Input: part model. Units: mm. Frame: model coordinates. Face numbers are marked on the shaded views. A direction names the side the tool comes from. Round coordinates to 2 decimals unless told otherwise and drop trailing zeros. Loops run counter-clockwise (first coordinate to the right, second up) from the corner with the lowest first, then second, coordinate; pieces in that order, holes last. Notation, with made-up numbers: (88.25, -4) - (119.25, -4) arc R16 ccw to (119.25, 17) - close; hole circle Ø1 at (29, 45). An arc over 180 degrees is marked (long way). Write each question's results on one line, items separated by ' | '.
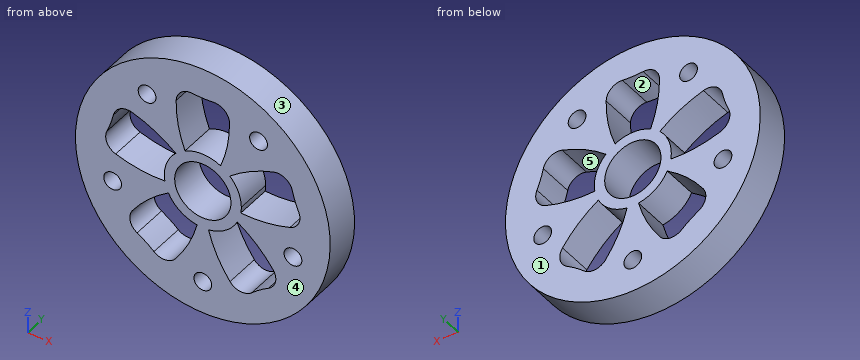
from build123d import *

# Parameters (mm, degrees)
SKETCH_1_R               = 43
SKETCH_1_R_2             = 9.5
SKETCH_1_R_3             = 3
EXTRUDE_1_DEPTH          = 12
CUT_EXTRUDE_1_DEPTH      = 62.983868869
CUT_EXTRUDE_1_DEPTH_BACK = 62.983868869


with BuildPart() as part:
    # 草图1 → 凸台-拉伸1 (new body)
    with BuildSketch(Plane(origin=(0, 0, 0), x_dir=(1, 0, 0), z_dir=(0, 1, 0))):
        with Locations(Location((0, 0, 0), (0, 0, 270))):
            Circle(SKETCH_1_R)
        with Locations(Location((0, 0, 0), (0, 0, 270))):
            Circle(SKETCH_1_R_2, mode=Mode.SUBTRACT)
        with Locations(Location((0, 32, 0), (0, 0, 270))):
            Circle(SKETCH_1_R_3, mode=Mode.SUBTRACT)
        with Locations(Location((30.433808521, 9.88854382, 0), (0, 0, 270))):
            Circle(SKETCH_1_R_3, mode=Mode.SUBTRACT)
        with Locations(Location((18.809128073, -25.88854382, 0), (0, 0, 270))):
            Circle(SKETCH_1_R_3, mode=Mode.SUBTRACT)
        with Locations(Location((-18.809128073, -25.88854382, 0), (0, 0, 270))):
            Circle(SKETCH_1_R_3, mode=Mode.SUBTRACT)
        with Locations(Location((-30.433808521, 9.88854382, 0), (0, 0, 270))):
            Circle(SKETCH_1_R_3, mode=Mode.SUBTRACT)
    extrude(amount=EXTRUDE_1_DEPTH)

    # 草图2 → 切除-拉伸1 (cut, two sides: drawn at the far end of the back side and taken through both)
    with BuildSketch(Plane(origin=(0, 0, 0), x_dir=(1, 0, 0), z_dir=(0, 1, 0)).offset(-CUT_EXTRUDE_1_DEPTH_BACK)):
        with BuildLine():
            ThreePointArc((-23.848620344, -17.211397152), (-16.091180112, -13.964625454), (-9.114016839, -9.270096928))
            ThreePointArc((-9.114016839, -9.270096928), (-12.363734712, -4.017220927), (-12.822220771, 2.142581267))
            ThreePointArc((-12.822220771, 2.142581267), (-21.226239066, 1.839460951), (-29.410544568, -0.093554533))
            ThreePointArc((-29.410544568, -0.093554533), (-32.369922784, -2.815813731), (-32.36785177, -6.83683478))
            ThreePointArc((-32.36785177, -6.83683478), (-31.119439219, -10.111318738), (-30.204732809, -13.494230394))
            ThreePointArc((-30.204732809, -13.494230394), (-27.842911423, -16.748522069), (-23.848620344, -17.211397152))
        make_face()
        with BuildLine():
            ThreePointArc((8.999382438, -28), (8.308699922, -19.618928286), (6, -11.532562595))
            ThreePointArc((6, -11.532562595), (0, -13), (-6, -11.532562595))
            ThreePointArc((-6, -11.532562595), (-8.308699922, -19.618928286), (-8.999382438, -28))
            ThreePointArc((-8.999382438, -28), (-7.324858249, -31.655760291), (-3.5, -32.896354479))
            ThreePointArc((-3.5, -32.896354479), (0, -32.720914778), (3.5, -32.896354479))
            ThreePointArc((3.5, -32.896354479), (7.324858249, -31.655760291), (8.999382438, -28))
        make_face()
        with BuildLine():
            ThreePointArc((12.822220771, 2.142581267), (12.955478957, 1.074972086), (13, 0))
            ThreePointArc((13, 0), (11.989208041, -5.025822375), (9.114016839, -9.270096928))
            ThreePointArc((9.114016839, -9.270096928), (16.091180112, -13.964625454), (23.848620344, -17.211397152))
            ThreePointArc((23.848620344, -17.211397152), (27.842911423, -16.748522069), (30.204732809, -13.494230394))
            ThreePointArc((30.204732809, -13.494230394), (31.119439219, -10.111318738), (32.36785177, -6.83683478))
            ThreePointArc((32.36785177, -6.83683478), (32.369922784, -2.815813731), (29.410544568, -0.093554533))
            ThreePointArc((29.410544568, -0.093554533), (21.226239066, 1.839460951), (12.822220771, 2.142581267))
        make_face()
        with BuildLine():
            ThreePointArc((1.924568248, 12.856750642), (7.64120828, 10.517220927), (11.632772181, 5.803327614))
            ThreePointArc((11.632772181, 5.803327614), (18.25359615, 10.988315115), (23.738640395, 17.362771566))
            ThreePointArc((23.738640395, 17.362771566), (24.532723854, 21.304604391), (22.167551497, 24.556461444))
            ThreePointArc((22.167551497, 24.556461444), (19.232871148, 26.471776127), (16.504432537, 28.67095821))
            ThreePointArc((16.504432537, 28.67095821), (12.680854244, 29.915491699), (9.177333733, 27.942180119))
            ThreePointArc((9.177333733, 27.942180119), (4.809837274, 20.755777674), (1.924568248, 12.856750642))
        make_face()
        with BuildLine():
            ThreePointArc((-11.632772181, 5.803327614), (-7.64120828, 10.517220927), (-1.924568248, 12.856750642))
            ThreePointArc((-1.924568248, 12.856750642), (-4.809837274, 20.755777674), (-9.177333733, 27.942180119))
            ThreePointArc((-9.177333733, 27.942180119), (-12.680854244, 29.915491699), (-16.504432537, 28.67095821))
            ThreePointArc((-16.504432537, 28.67095821), (-19.232871148, 26.471776127), (-22.167551497, 24.556461444))
            ThreePointArc((-22.167551497, 24.556461444), (-24.532723854, 21.304604391), (-23.738640395, 17.362771566))
            ThreePointArc((-23.738640395, 17.362771566), (-18.25359615, 10.988315115), (-11.632772181, 5.803327614))
        make_face()
    extrude(amount=CUT_EXTRUDE_1_DEPTH + CUT_EXTRUDE_1_DEPTH_BACK, mode=Mode.SUBTRACT)


solid = part.part
1. Section query C-C, the plane z = 16. Output: boundary loops of the cut face in (x, y).
Answer:
outline: (-39.91, 0) - (-28.82, 0) - (-28.82, 12) - (-39.91, 12) - close; (-20.43, 0) - (-7.49, 0) - (-7.49, 12) - (-20.43, 12) - close; (7.49, 0) - (20.43, 0) - (20.43, 12) - (7.49, 12) - close; (28.82, 0) - (39.91, 0) - (39.91, 12) - (28.82, 12) - close
2. Section query A-A, the plane x = 0. Output: boundary loops of the cut face in (y, z).
Answer:
outline: (0, -43) - (12, -43) - (12, -35) - (0, -35) - close; (0, -29) - (12, -29) - (12, -9.5) - (0, -9.5) - close; (0, 9.5) - (12, 9.5) - (12, 13) - (0, 13) - close; (0, 32.72) - (12, 32.72) - (12, 43) - (0, 43) - close
3. Set-up query: the marked faces 1 and 2. Return all of +Z, -Z, +X, -X, +Y, -Y with unobstructed straight access to the full face (end or side cutting, diameter ignored); none if empty.
Answer:
face 1: +Z, -Z, +X, -X, +Y | face 2: +Y, -Y
4. Mould query, pull axis X, two halves, no side actions, for the marked faces 3, 4 and 5. Classes: pulls with the +X half, pulls with the -X half, needs draft (parallel to the pull), parting line crosses it, or undercut.
Answer:
face 3: parting line crosses it | face 4: needs draft | face 5: undercut
5. Section query B-B, the plane z = -32. Output: boundary loops of the cut face in (x, y).
Answer:
outline: (-28.72, 0) - (-3, 0) - (-3, 12) - (-28.72, 12) - close; (3, 0) - (28.72, 0) - (28.72, 12) - (3, 12) - close
6. Section query D-D, the plane y = 1. Count the separate pieces of the cut face and the enclosed holes in it, plus the area to 3 significant figures.
Answer:
separate pieces: 1 | enclosed holes: 11 | area: 3,730 mm^2
7. Line query: line 1 (X direction, y = 7.5, z = 5.5) (3 decimals); line 2 (X direction, y = 10.5, z = -29.5); line 3 (X direction, y = 9.5, z = 11). Output: solid intervals per line, ascending. Write a range as [from, to].
Answer:
line 1: [-42.647, -32.745], [-11.779, -7.746], [7.746, 11.779], [32.745, 42.647] | line 2: [-31.28, -15.23], [-11.12, -1.66], [1.66, 11.12], [15.23, 31.28] | line 3: [-41.57, -30.84], [-11.36, 11.36], [30.84, 41.57]
8. Contact query for flat-ended pins moving along their axis: pin 1 (6 mm diameter, centred on y = 6, z = -25, fed in from -X); pin 2 (2 mm diameter, centred on x = 30.5, y = 5, fed in from -Z) (3 decimals); pin 3 (3.5 mm diameter, centred on x = 30.43, z = -9.89, fed in from -Y) (3 decimals); pin 4 (5 mm diameter, centred on x = -24.5, y = 10.5, fed in from +Z). Output: stop coordinate, or through.
Answer:
pin 1: x = -36.95 | pin 2: z = -31.285 | pin 3: through | pin 4: z = 36.95
